CAD build for the part. Positions are in the model's coordinates, mm. Give positions to 0.01 mm unless a question says otherwise; leave off trailing zeros. Loops run counter-clockwise (first coordinate to the right, second up) from the corner with the lowest first, then second, coordinate; pieces in that order, holes last.
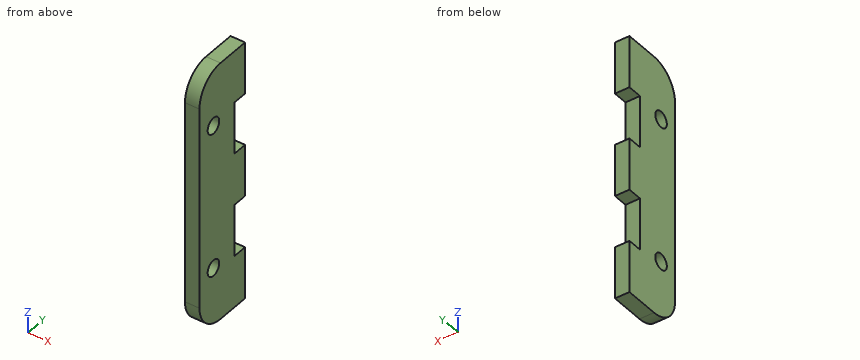
```python
from build123d import *

# Parameters (mm, degrees)
SKETCH1_R           = 1.65
BOSS_EXTRUDE1_DEPTH = 3


with BuildPart() as part:
    # Sketch1 → Boss-Extrude1 (new body)
    with BuildSketch(Plane(origin=(0, 0, 0), x_dir=(0, 0, -1), z_dir=(1, 0, 0))):
        with BuildLine():
            Line((21, -6.5), (-21, -6.5))
            ThreePointArc((-21, -6.5), (-25.242640687, -4.742640687), (-27, -0.5))
            Line((-27, -0.5), (-27, 6.5))
            Line((-27, 6.5), (-16.2, 6.5))
            Line((-16.2, 6.5), (-16.2, 3.5))
            Line((-16.2, 3.5), (-5.4, 3.5))
            Line((-5.4, 3.5), (-5.4, 6.5))
            Line((-5.4, 6.5), (5.4, 6.5))
            Line((5.4, 6.5), (5.4, 3.5))
            Line((5.4, 3.5), (16.2, 3.5))
            Line((16.2, 3.5), (16.2, 6.5))
            Line((16.2, 6.5), (27, 6.5))
            Line((27, 6.5), (27, -0.5))
            ThreePointArc((27, -0.5), (25.242640687, -4.742640687), (21, -6.5))
        make_face()
        with Locations((-15, -2.509032308)):
            Circle(SKETCH1_R, mode=Mode.SUBTRACT)
        with Locations((15, -2.509032308)):
            Circle(SKETCH1_R, mode=Mode.SUBTRACT)
    extrude(amount=BOSS_EXTRUDE1_DEPTH)


solid = part.part
```
1. Saw through at D-D, the plane z = 11. List the corners of the cut face in (x, y).
Responses:
outline: (0, -6.5) - (3, -6.5) - (3, 3.5) - (0, 3.5) - close
2. Drop a flat-ended pin along its axis: pin 1 (0.9 mm diameter, centred on x = 1.5, z = 11, fed in from +Y). Give the stop position or say it passes through.
Responses:
pin 1: stops at y = 3.5
3. Probe line 1 along Z through (x, y) = (1.6, 5.5); line 2 along Z through (x, y) = (0.25, -2); line 3 along Y through (x, z) = (2, 15). List the from-to ranges inside material, lowest first.
Responses:
line 1: z = -27 to -16.2, -5.4 to 5.4, 16.2 to 27
line 2: z = -26.81 to -16.57, -13.43 to 13.43, 16.57 to 26.81
line 3: y = -6.5 to -4.16, -0.86 to 3.5
4. Saw through at C-C, the plane x = 1.25. List the corners of the cut face in (y, z).
Responses:
outline: (-6.5, -21) arc R6 ccw to (-0.5, -27) - (6.5, -27) - (6.5, -16.2) - (3.5, -16.2) - (3.5, -5.4) - (6.5, -5.4) - (6.5, 5.4) - (3.5, 5.4) - (3.5, 16.2) - (6.5, 16.2) - (6.5, 27) - (-0.5, 27) arc R6 ccw to (-6.5, 21) - close; hole circle Ø3.3 at (-2.51, -15); hole circle Ø3.3 at (-2.51, 15)
5. Saw through at B-B, the plane y = 5.5. List the corners of the cut face in (x, z), and give its area (3 significant figures).
Responses:
outline: (0, -27) - (3, -27) - (3, -16.2) - (0, -16.2) - close; (0, -5.4) - (3, -5.4) - (3, 5.4) - (0, 5.4) - close; (0, 16.2) - (3, 16.2) - (3, 27) - (0, 27) - close
area: 97.2 mm2
6. Saw through at A-A, the plane z = -15. List the corners of the cut face in (x, y), and give its area (3 significant figures).
Responses:
outline: (0, -6.5) - (3, -6.5) - (3, -4.16) - (0, -4.16) - close; (0, -0.86) - (3, -0.86) - (3, 3.5) - (0, 3.5) - close
area: 20.1 mm2
